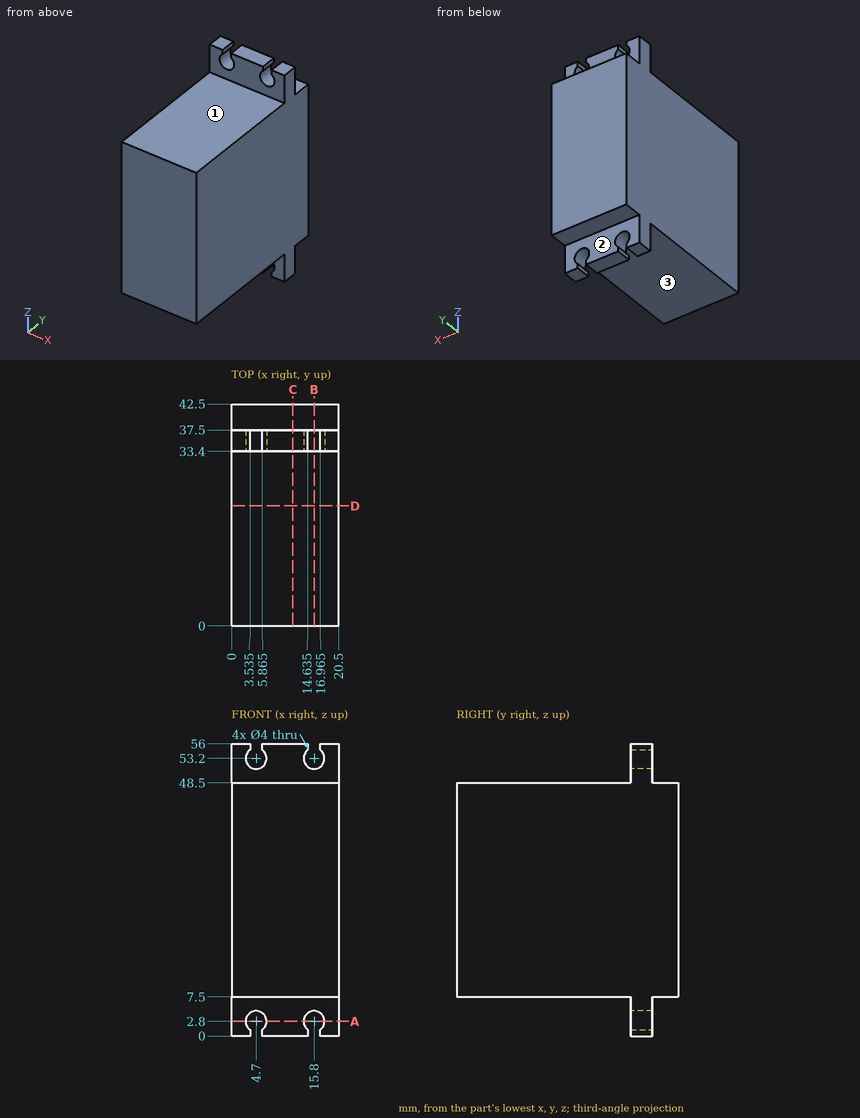
Geometry: see drawing. Coordinates: mm, zero at the bounding-box minimum. A direction names the side the tool comes from. Give positions to 0.01 mm unless a question says otherwise; leave off trailing zeros. Write each loop counter-clockwise with the first axis right and the second up, starting at its lowest first coordinate (ties: lowest second). Pieces come first, ordered by that corner, then holes. Notation, with made-up numbers: (81.25, 4.5) - (101.25, 4.5) arc R12 cw to (101.25, 17.5) - close; hole circle Ø10 at (50, 38). An arc over 180 degrees is marked (long way). Return JSON: item names as keys, results as strings. Group by question number.
1) Section A-A on z = 2.8. Return the cut outline in (x, y).
2) Section C-C on x = 11.75. Return the cut outline in (y, z).
3) Line query: line 1 (X direction, y = 35.5, z = 53.2); line 2 (Y direction, x = 1.75, z = 3); line 3 (Z direction, x = 6.5, y = 25). Output: solid intervals per line, ascending.
4) First-contact query: P1, Ø1.3, axis at y = 35.5, z = 55.5, coming from the -X side; P2, Ø6.5, axis at x = 4.7, z = 53.2, coming from the -Y side; P3, Ø1, axis at x = 13.5, y = 29.5, coming from the +Z side; P4, Ø2.5, axis at x = 7, y = 41, coming from the -Z side. Flat tips, straight axial feed; report the tip coordinate or a pass-through.
5) Section D-D on y = 23. Return the cut outline in (x, z).
6) Section B-B on x = 15.8. Return the cut outline in (y, z).
7) Set-up query: the marked faces 1, 2 and 3. Return all of +Z, -Z, +X, -X, +Y, -Y with unobstructed straight access to the full face (end or side cutting, diameter ignored); none if empty.
Filled in:
{
 "1": {"outline": "(0, 33.4) - (2.7, 33.4) - (2.7, 37.5) - (0, 37.5) - close; (6.7, 33.4) - (13.8, 33.4) - (13.8, 37.5) - (6.7, 37.5) - close; (17.8, 33.4) - (20.5, 33.4) - (20.5, 37.5) - (17.8, 37.5) - close"},
 "2": {"outline": "(0, 7.5) - (33.4, 7.5) - (33.4, 0) - (37.5, 0) - (37.5, 7.5) - (42.5, 7.5) - (42.5, 48.5) - (37.5, 48.5) - (37.5, 56) - (33.4, 56) - (33.4, 48.5) - (0, 48.5) - close"},
 "3": {"line 1": "x = 0 to 2.7, 6.7 to 13.8, 17.8 to 20.5", "line 2": "y = 33.4 to 37.5", "line 3": "z = 7.5 to 48.5"},
 "4": {"P1": "stops at x = 0", "P2": "stops at y = 33.4", "P3": "stops at z = 48.5", "P4": "stops at z = 7.5"},
 "5": {"outline": "(0, 7.5) - (20.5, 7.5) - (20.5, 48.5) - (0, 48.5) - close"},
 "6": {"outline": "(0, 7.5) - (33.4, 7.5) - (33.4, 4.8) - (37.5, 4.8) - (37.5, 7.5) - (42.5, 7.5) - (42.5, 48.5) - (37.5, 48.5) - (37.5, 51.2) - (33.4, 51.2) - (33.4, 48.5) - (0, 48.5) - close"},
 "7": {"face 1": "+Z, +X, -X, -Y", "face 2": "-Z, +X, -X, +Y", "face 3": "-Z, +X, -X, -Y"}
}
